Source: CAD feature listing. Evaluate the final solid. Frame: model axes, mm. A direction names the side the tool comes from. Coordinates: 2 decimals unless noted, no trailing zeros. Loops run counter-clockwise (first coordinate to the right, second up) from the corner with the lowest first, then second, coordinate; pieces in that order, holes last. Notation, with made-up numbers: M 83.5,22.5 L 122.5,22.5 A28 cw 122.5,61.5 Z; hole C -28.75,50 d7. An arc over 180 degrees is marked long. One line per question, with ' | ' between items. Start each with the question number.
1. Access query for faces 4 (the flat face through (68.89, -43.17, 1.52)), 5 (the flat face through (-43.17, -68.89, 1.52)), 6 (the flat face through (43.17, 68.89, 1.52)), 7 (the flat face through (-25.7, -13.9, 1.5)), 8 (the flat face through (78.46, 46.64, 1.52)). Directions: +Z, -Z, +X, -X, +Y, -Y. A direction counts if a zero-diameter tool reaches every point of the face in a straight line with its end or side. Return the directions, or none.
2. Mould query, pull axis X, two halves, no side actions, for faces 1 (the flat face through (-46.64, 78.46, 1.52)), 2 (the flat face through (-25.6, 14, 1.5)), 3 (the cylindrical face through (-0.782, -99.997, 1.479)). Classes: pulls with the +X half, pulls with the -X half, needs draft (parallel to the pull), parting line crosses it, or undercut.
3. Ray query, probe 1 along X at (y, z) = (0, 1.15); probe 2 along X at (y, z) = (-38.5, 1); probe 3 along Y at (x, z) = (5, 1.5). Return the intervals inside material, ascending.
4. Section query B-B, the plane y = -79.5. Output: boundary loops of the cut face in (x, z).
5. Pin query (flat end, axial travel): P1, Ø1.5, axis at y = 25.5, z = 0.5, coming from the +X side; P2, Ø2.5, axis at x = -4.5, y = 47.8, coming from the +Z side; P3, Ø10, axis at x = 66.5, y = 12, coming from the -Z side; P4, Ø0.9, axis at x = 41.5, z = 1, coming from the -Y side. Return the tip coordinate at first contact, or that it passes through.
6. Section query A-A, the plane z = 2.3. State how many separate pieces and enclosed holes the cut face has, and give its area (3 significant figures).
```python
from build123d import *

# Parameters (mm, degrees)
CROQUIS1_R              = 100
SALIENTE_EXTRUIR1_DEPTH = 3
CROQUIS3_R              = 110
CORTAR_EXTRUIR1_DEPTH   = 3
REDONDEO1_R             = 10
CORTAR_EXTRUIR2_DEPTH   = 10
CORTAR_EXTRUIR3_DEPTH   = 10
CROQUIS8_R              = 1.5
CROQUIS8_R_2            = 1.502317269
CROQUIS8_R_3            = 2
CORTAR_EXTRUIR4_DEPTH   = 10
CROQUIS9_R              = 1.5
CROQUIS9_W              = 4.5
CROQUIS9_H              = 7.5
CROQUIS9_W_2            = 7.5
CROQUIS9_H_2            = 4.5
CORTAR_EXTRUIR5_DEPTH   = 10
CORTAR_EXTRUIR6_DEPTH   = 3


with BuildPart() as part:
    # Croquis1 → Saliente-Extruir1 (new body)
    with BuildSketch(Plane.XY):
        Circle(CROQUIS1_R)
    extrude(amount=SALIENTE_EXTRUIR1_DEPTH)

    # Croquis3 → Cortar-Extruir1 (cut)
    with BuildSketch(Plane.XY.offset(3)):
        with Locations((190, 0)):
            Circle(CROQUIS3_R)
    extrude(amount=-CORTAR_EXTRUIR1_DEPTH, mode=Mode.SUBTRACT)

    # Redondeo1
    redondeo1_edges = [part.edges().sort_by_distance(p)[0] for p in [
        (89.473684211, -44.659375654, 1.5),
        (89.473684211, 44.659375654, 1.5),
    ]]
    fillet(redondeo1_edges, radius=REDONDEO1_R)

    # Croquis5 → Cortar-Extruir2 (cut)
    with BuildSketch(Plane.XY.offset(3)):
        Polygon((-29.69848481, -9.899494937), (-9.899494937, -29.69848481), (-64.346717088, -84.145706961), (-84.145706961, -64.346717088), align=None)
        Polygon((-9.899494937, 29.69848481), (-29.69848481, 9.899494937), (-84.145706961, 64.346717088), (-64.346717088, 84.145706961), align=None)
        Polygon((29.69848481, 9.899494937), (9.899494937, 29.69848481), (64.346717088, 84.145706961), (84.145706961, 64.346717088), align=None)
        Polygon((9.899494937, -29.69848481), (29.69848481, -9.899494937), (84.145706961, -64.346717088), (64.346717088, -84.145706961), align=None)
    extrude(amount=-CORTAR_EXTRUIR2_DEPTH, mode=Mode.SUBTRACT)

    # Croquis7 → Cortar-Extruir3 (cut)
    with BuildSketch(Plane.XY.offset(3)):
        Polygon((-71.939339828, -40.119534675), (-40.119534675, -71.939339828), (-57.090097423, -88.909902577), (-88.909902577, -57.090097423), align=None)
        Polygon((-40.119534675, 71.939339828), (-71.939339828, 40.119534675), (-88.909902577, 57.090097423), (-57.090097423, 88.909902577), align=None)
        Polygon((71.939339828, 40.119534675), (40.119534675, 71.939339828), (57.090097423, 88.909902577), (88.909902577, 57.090097423), align=None)
        Polygon((40.119534675, -71.939339828), (71.939339828, -40.119534675), (88.909902577, -57.090097423), (57.090097423, -88.909902577), align=None)
        Polygon((-21.566756826, -18.03122292), (-18.03122292, -21.566756826), (-14.495689014, -18.03122292), (-18.03122292, -14.495689014), align=None)
        Polygon((-21.566756826, 18.03122292), (-18.03122292, 14.495689014), (-14.495689014, 18.03122292), (-18.03122292, 21.566756826), align=None)
        Polygon((18.03122292, 21.566756826), (14.495689014, 18.03122292), (18.03122292, 14.495689014), (21.566756826, 18.03122292), align=None)
        Polygon((21.566756826, -18.03122292), (18.03122292, -14.495689014), (14.495689014, -18.03122292), (18.03122292, -21.566756826), align=None)
    extrude(amount=-CORTAR_EXTRUIR3_DEPTH, mode=Mode.SUBTRACT)

    # Croquis8 → Cortar-Extruir4 (cut)
    with BuildSketch(Plane.XY.offset(3)):
        with Locations((-64.762205999, 40.904423202)):
            Circle(CROQUIS8_R)
        with Locations((-48.852303422, 24.994520625)):
            Circle(CROQUIS8_R_2)
        with Locations((-24.994520625, 48.852303422)):
            Circle(CROQUIS8_R)
        with Locations((-40.904423202, 64.762205999)):
            Circle(CROQUIS8_R)
        with Locations((64.762205999, 40.904423202)):
            Circle(CROQUIS8_R)
        with Locations((48.852303422, 24.994520625)):
            Circle(CROQUIS8_R)
        with Locations((24.994520625, 48.852303422)):
            Circle(CROQUIS8_R_2)
        with Locations((40.904423202, 64.762205999)):
            Circle(CROQUIS8_R)
        with Locations((40.904423202, -64.762205999)):
            Circle(CROQUIS8_R)
        with Locations((24.994520625, -48.852303422)):
            Circle(CROQUIS8_R)
        with Locations((48.852303422, -24.994520625)):
            Circle(CROQUIS8_R_2)
        with Locations((64.762205999, -40.904423202)):
            Circle(CROQUIS8_R)
        with Locations((-64.762205999, -40.904423202)):
            Circle(CROQUIS8_R)
        with Locations((-48.852303422, -24.994520625)):
            Circle(CROQUIS8_R)
        with Locations((-24.994520625, -48.852303422)):
            Circle(CROQUIS8_R_2)
        with Locations((-40.904423202, -64.762205999)):
            Circle(CROQUIS8_R)
        with Locations((0, 92)):
            Circle(CROQUIS8_R_3)
        with Locations((0, -92)):
            Circle(CROQUIS8_R_3)
        with Locations((72, 31.694913472)):
            Circle(CROQUIS8_R_3)
        with Locations((72, -31.694913472)):
            Circle(CROQUIS8_R_3)
        with Locations((-85, -30)):
            Circle(CROQUIS8_R_3)
        with Locations((-85, 30)):
            Circle(CROQUIS8_R_3)
    extrude(amount=-CORTAR_EXTRUIR4_DEPTH, mode=Mode.SUBTRACT)

    # Croquis9 → Cortar-Extruir5 (cut)
    with BuildSketch(Plane.XY.offset(3)):
        with Locations((73.1, -4.5)):
            Circle(CROQUIS9_R)
        with Locations((35.9, 4.5)):
            Circle(CROQUIS9_R)
        with Locations((73.1, 4.5)):
            Circle(CROQUIS9_R)
        with Locations((35.9, -4.5)):
            Circle(CROQUIS9_R)
        with Locations((-91.190074744, 4.5)):
            Circle(CROQUIS9_R)
        with Locations((-91.190074744, -4.5)):
            Circle(CROQUIS9_R)
        with Locations((-53.990074744, 4.5)):
            Circle(CROQUIS9_R)
        with Locations((-53.990074744, -4.5)):
            Circle(CROQUIS9_R)
        with Locations((-4.5, 85)):
            Circle(CROQUIS9_R)
        with Locations((4.5, 85)):
            Circle(CROQUIS9_R)
        with Locations((-4.5, 47.8)):
            Circle(CROQUIS9_R)
        with Locations((4.5, 47.8)):
            Circle(CROQUIS9_R)
        with Locations((-4.5, -47.8)):
            Circle(CROQUIS9_R)
        with Locations((4.5, -47.8)):
            Circle(CROQUIS9_R)
        with Locations((4.5, -85)):
            Circle(CROQUIS9_R)
        with Locations((-4.5, -85)):
            Circle(CROQUIS9_R)
        with Locations((39.85, 0)):
            Rectangle(CROQUIS9_W, CROQUIS9_H)
        with Locations((0, -51.75)):
            Rectangle(CROQUIS9_W_2, CROQUIS9_H_2)
        with Locations((-57.940074744, 0)):
            Rectangle(CROQUIS9_W, CROQUIS9_H)
        with Locations((0, 51.75)):
            Rectangle(CROQUIS9_W_2, CROQUIS9_H_2)
    extrude(amount=-CORTAR_EXTRUIR5_DEPTH, mode=Mode.SUBTRACT)

    # Croquis10 → Cortar-Extruir6 (cut)
    with BuildSketch(Plane.XY.offset(3)):
        with BuildLine():
            Line((-4.5, 49.3), (-4.5, 55.3))
            Line((-4.5, 55.3), (4.5, 55.3))
            Line((4.5, 55.3), (4.5, 49.3))
            ThreePointArc((4.5, 49.3), (3.439339828, 48.860660172), (3, 47.8))
            Line((3, 47.8), (-3, 47.8))
            ThreePointArc((-3, 47.8), (-3.439339828, 48.860660172), (-4.5, 49.3))
        make_face()
        with BuildLine():
            Line((43.4, 4.5), (37.4, 4.5))
            ThreePointArc((37.4, 4.5), (36.960660172, 3.439339828), (35.9, 3))
            Line((35.9, 3), (35.9, -3))
            ThreePointArc((35.9, -3), (36.960660172, -3.439339828), (37.4, -4.5))
            Line((37.4, -4.5), (43.4, -4.5))
            Line((43.4, -4.5), (43.4, 4.5))
        make_face()
        with BuildLine():
            ThreePointArc((3, -47.8), (3.439339828, -48.860660172), (4.5, -49.3))
            Line((4.5, -49.3), (4.5, -55.3))
            Line((4.5, -55.3), (-4.5, -55.3))
            Line((-4.5, -55.3), (-4.5, -49.3))
            ThreePointArc((-4.5, -49.3), (-3.439339828, -48.860660172), (-3, -47.8))
            Line((-3, -47.8), (3, -47.8))
        make_face()
        with BuildLine():
            Line((-61.490074744, -4.5), (-55.490074744, -4.5))
            ThreePointArc((-55.490074744, -4.5), (-55.050734915, -3.439339828), (-53.990074744, -3))
            Line((-53.990074744, -3), (-53.990074744, 3))
            ThreePointArc((-53.990074744, 3), (-55.050734915, 3.439339828), (-55.490074744, 4.5))
            Line((-55.490074744, 4.5), (-61.490074744, 4.5))
            Line((-61.490074744, 4.5), (-61.490074744, -4.5))
        make_face()
    extrude(amount=-CORTAR_EXTRUIR6_DEPTH, mode=Mode.SUBTRACT)


solid = part.part
```
Taken from the geometry:
1) face 4: +Z, -Z, -Y | face 5: +Z, -Z, -X | face 6: +Z, -Z, +X | face 7: +Z, -Z | face 8: +Z, -Z, +Y
2) face 1: pulls with the -X half | face 2: undercut | face 3: parting line crosses it
3) probe 1: -100 to -61.49, -53.99 to 35.9, 43.4 to 80 | probe 2: -92.29 to -58.3, -18.7 to 18.7, 58.3 to 86.96 | probe 3: -99.87 to -86.41, -83.59 to -49.21, -46.39 to 46.39, 49.21 to 83.59, 86.41 to 99.87
4) outline: M -47.68,0 L 47.68,0 L 47.68,3 L -47.68,3 Z
5) P1: x = 83.18 | P2: through | P3: z = 0 | P4: y = -91.19
6) separate pieces: 1 | enclosed holes: 34 | area: 20,200 mm^2
